CAD build for the part. Positions are in the model's coordinates, mm. Face numbers are marked on the shaded views. A direction names the side the tool comes from. Round coordinates to 2 decimals unless told otherwise and drop trailing zeros. Order: outer loops, then holes, each group sorted by start corner. A loop starts at its lowest first (then second) coordinate and runs counter-clockwise, first axis right, second up. Notation, with made-up numbers: (20.25, 42.25) - (78.25, 42.25) arc R6 cw to (78.25, 52.25) - close; hole circle Ø11 at (27.5, 58). An arc over 180 degrees is marked (long way). Write item = value, one per line.
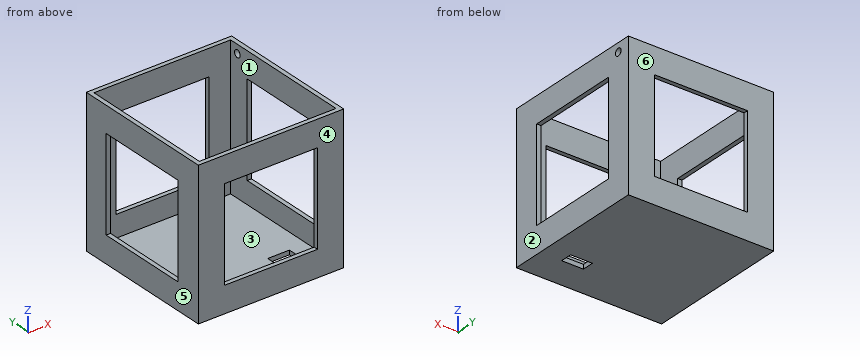
Autodesk Fusion 360 part; units mm, degrees
sketch "Sketch1" plane through (0, 0, 0) normal (0, 0, 1) x (1, 0, 0)
  line L0 (-50, 50) -> (60, 50)
  line L1 (60, 50) -> (60, -50)
  line L2 (60, -50) -> (-50, -50)
  line L3 (-50, -50) -> (-50, 50)
sketch "Sketch8" plane through (0, 0, 0) normal (0, 0, 1) x (1, 0, 0)
  line L0 (-50, 50) -> (50, 50)
  line L1 (50, 50) -> (50, -50)
  line L2 (50, -50) -> (-50, -50)
  line L3 (-50, -50) -> (-50, 50)
  line L4 (-50, 50) -> (50, -50) construction
  line L5 (50, 50) -> (-50, -50) construction
  dimension "d15" = 100
  dimension "d16" = 100
extrude "Extrude3" add sketch "Sketch8" along normal blind 100
sketch "Sketch9" plane through (0, 0, 100) normal (0, 0, 1) x (-1, 0, 0)
  line L0 (50, 50) -> (-50, 50)
  line L1 (-50, 50) -> (-50, -50)
  line L2 (-50, -50) -> (50, -50)
  line L3 (50, -50) -> (50, 50)
shell "Shell2" thickness 3 removed faces 1 at (-16.6667, 16.6667, 100)
sketch "Sketch10" plane through (50, 0, 0) normal (1, 0, 0) x (0, 1, 0)
  line L0 (-50, 0) -> (50, 0)
  line L1 (50, 0) -> (50, 100)
  line L2 (50, 100) -> (-50, 100)
  line L3 (-50, 100) -> (-50, 0)
  line L4 (32.2521, 82.1964) -> (-31.7479, 82.1964)
  line L5 (-31.7479, 82.1964) -> (-31.7479, 18.1964)
  line L6 (-31.7479, 18.1964) -> (32.2521, 18.1964)
  line L7 (32.2521, 18.1964) -> (32.2521, 82.1964)
  line L8 (32.2521, 82.1964) -> (-31.7479, 18.1964) construction
  line L9 (-31.7479, 82.1964) -> (32.2521, 18.1964) construction
  point P0 (0.2521, 50.1964)
  dimension "d20" = 64
  dimension "d21" = 64
extrude "Extrude4" cut sketch "Sketch10" against normal through all contours L4 L5 L6 L7
sketch "Sketch11" plane through (0, -50, 0) normal (0, -1, 0) x (1, 0, 0)
  line L0 (-50, 0) -> (50, 0)
  line L1 (50, 0) -> (50, 100)
  line L2 (50, 100) -> (-50, 100)
  line L3 (-50, 100) -> (-50, 0)
  line L4 (-32, 82) -> (32, 82)
  line L5 (32, 82) -> (32, 18)
  line L6 (32, 18) -> (-32, 18)
  line L7 (-32, 18) -> (-32, 82)
  line L8 (-32, 82) -> (32, 18) construction
  line L9 (32, 82) -> (-32, 18) construction
  point P0 (0, 50)
  dimension "d23" = 64
  dimension "d24" = 64
extrude "Extrude5" cut sketch "Sketch11" against normal blind 110 contours L4 L5 L6 L7
sketch "Sketch12" plane through (0, 0, 0) normal (0, 0, 1) x (1, 0, 0)
  line L0 (35.1289, -20.848) -> (20.1289, -20.848)
  line L1 (20.1289, -20.848) -> (20.1289, -28.848)
  line L2 (20.1289, -28.848) -> (35.1289, -28.848)
  line L3 (35.1289, -28.848) -> (35.1289, -20.848)
  dimension "d27" = 15
  dimension "d28" = 8
extrude "Extrude6" cut sketch "Sketch12" along normal blind 3
sketch "Sketch13" plane through (50, 0, 0) normal (1, 0, 0) x (0, 1, 0)
  line L0 (32.2521, 18.1964) -> (-31.7479, 18.1964)
  line L1 (-31.7479, 18.1964) -> (-31.7479, 82.1964)
  line L2 (-31.7479, 82.1964) -> (32.2521, 82.1964)
  line L3 (32.2521, 82.1964) -> (32.2521, 18.1964)
  line L4 (-50, 0) -> (50, 0)
  line L5 (50, 0) -> (50, 100)
  line L6 (50, 100) -> (-50, 100)
  line L7 (-50, 100) -> (-50, 0)
  circle A0 centre (41, 94) radius 2.5
  dimension "d31" = 5
extrude "Extrude7" cut sketch "Sketch13" against normal blind 3 contours A0
(1) Band-saw the part on D-D on z = 25. List the corners of the cut face in (x, y).
Solved:
outline = (-50, -50) - (-32, -50) - (-32, -47) - (-47, -47) - (-47, -31.75) - (-50, -31.75) - close; (-50, 32.25) - (-47, 32.25) - (-47, 47) - (-32, 47) - (-32, 50) - (-50, 50) - close; (32, -50) - (50, -50) - (50, -31.75) - (47, -31.75) - (47, -47) - (32, -47) - close; (32, 47) - (47, 47) - (47, 32.25) - (50, 32.25) - (50, 50) - (32, 50) - close
(2) Tool access for the marked faces 1 and 2: list every direction of +Z, -Z, +X, -X, +Y, -Y with a clear straight run to the whole face (end or side of a thin tool).
Solved:
face_1 = +Z
face_2 = +Z, -Z, +X, +Y, -Y
(3) Drop a flat-ended pin along its axis: pin 1 (6 mm diameter, centred on x = 22.5, y = 26.5, fed in from +Z). Give the stop position or say it passes through.
Solved:
pin_1 = 3
(4) Band-saw the part on B-B on y = -8.5. List the corners of the cut face in (x, z).
Solved:
outline = (-50, 0) - (50, 0) - (50, 18.2) - (47, 18.2) - (47, 3) - (-47, 3) - (-47, 18.2) - (-50, 18.2) - close; (-50, 82.2) - (-47, 82.2) - (-47, 100) - (-50, 100) - close; (47, 82.2) - (50, 82.2) - (50, 100) - (47, 100) - close
(5) Probe line 1 along Y through (x, z) = (35.5, 18); line 2 along Z through (x, y) = (49, 41). List the from-to ranges inside material, lowest first.
Solved:
line_1 = -50 to -47, 47 to 50
line_2 = 0 to 91.5, 96.5 to 100
(6) Band-saw the part on C-C on z = 14.5. List the corners of the cut face in (x, y).
Solved:
outline = (-50, -50) - (50, -50) - (50, 50) - (-50, 50) - close; hole (-47, -47) - (47, -47) - (47, 47) - (-47, 47) - close
(7) Pull direction Y, two halves, no side cores. Call the marked faces 3, 4, 5 and 6: released by +Y, released by -Y, zero draft, split by the parting line, or undercut.
Solved:
face_3 = undercut
face_4 = released by -Y
face_5 = zero draft
face_6 = released by +Y
(8) Band-saw the part on A-A on x = 15.5. List the corners of the cut face in (y, z).
Solved:
outline = (-50, 0) - (50, 0) - (50, 18) - (47, 18) - (47, 3) - (-47, 3) - (-47, 18) - (-50, 18) - close; (-50, 82) - (-47, 82) - (-47, 100) - (-50, 100) - close; (47, 82) - (50, 82) - (50, 100) - (47, 100) - close
